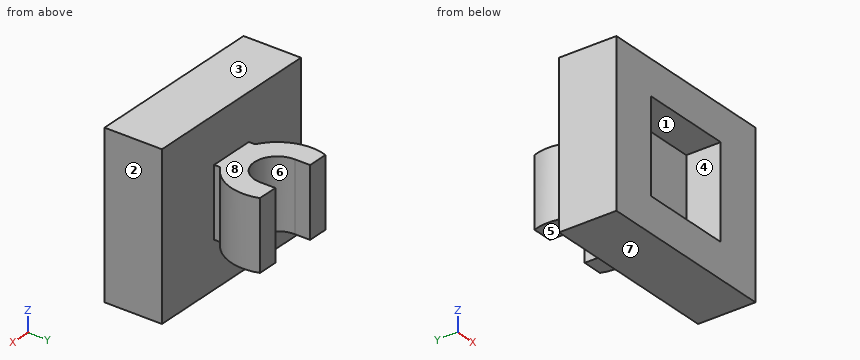
```python
from build123d import *

# Parameters (mm, degrees)
SKETCH1_W           = 10.16
SKETCH1_H           = 3.175
BOSS_EXTRUDE1_DEPTH = 4.445
BOSS_EXTRUDE2_DEPTH = 1.905
SKETCH3_OUTSIDE_W   = 15.162
SKETCH3_OUTSIDE_H   = 13.892
SKETCH3_OUTSIDE_W_2 = 10.16
SKETCH3_OUTSIDE_H_2 = 8.89
SKETCH3_OUTSIDE_W_3 = 5.08
SKETCH3_OUTSIDE_H_3 = 5.08
CUT_EXTRUDE1_DEPTH  = 1.905


with BuildPart() as part:
    # Sketch1 → Boss-Extrude1 (new body, symmetric)
    with BuildSketch(Plane.XY):
        with Locations((0, -1.5875)):
            Rectangle(SKETCH1_W, SKETCH1_H)
    extrude(amount=BOSS_EXTRUDE1_DEPTH, both=True)

    # Sketch2 → Boss-Extrude2 (add, symmetric)
    with BuildSketch(Plane.XY):
        with BuildLine():
            Line((-1.27, 2.54), (-1.27, 3.386666667))
            Line((-1.27, 3.386666667), (-2.394734966, 3.386666667))
            ThreePointArc((-2.394734966, 3.386666667), (-2.382785125, 1.660264217), (-1.27, 0.340295474))
            Line((-1.27, 0.340295474), (-1.27, 0))
            Line((-1.27, 0), (1.27, 0))
            Line((1.27, 0), (1.27, 0.340295474))
            ThreePointArc((1.27, 0.340295474), (2.382785125, 1.660264217), (2.394734966, 3.386666667))
            Line((2.394734966, 3.386666667), (1.27, 3.386666667))
            Line((1.27, 3.386666667), (1.27, 2.54))
            ThreePointArc((1.27, 2.54), (0, 1.27), (-1.27, 2.54))
        make_face()
    extrude(amount=BOSS_EXTRUDE2_DEPTH, both=True)

    # Sketch3 outside → Cut-Extrude1 (cut)
    with BuildSketch(Plane.XZ.offset(3.175)):
        Rectangle(SKETCH3_OUTSIDE_W, SKETCH3_OUTSIDE_H)
        Rectangle(SKETCH3_OUTSIDE_W_2, SKETCH3_OUTSIDE_H_2, mode=Mode.SUBTRACT)
        Rectangle(SKETCH3_OUTSIDE_W_3, SKETCH3_OUTSIDE_H_3)
    extrude(amount=-CUT_EXTRUDE1_DEPTH, mode=Mode.SUBTRACT)


solid = part.part
```
Can you work these out from the model? Positions are in its coordinate system, mm. Face numbers are marked on the shaded views. A direction names the side the tool comes from. Round coordinates to 2 decimals unless told otherwise and drop trailing zeros. Loops run counter-clockwise (first coordinate to the right, second up) from the corner with the lowest first, then second, coordinate; pieces in that order, holes last. Notation, with made-up numbers: (-8.75, -18) -> (31.25, -18) arc R19 cw to (31.25, -6) -> close; hole circle Ø5 at (79.25, 43). An arc over 180 degrees is marked (long way). Answer in a Markdown table with one row per item.
Item 1: Suppose I cut it at D-D, the plane y = 2.75. List the corners of the cut face in (x, z) for me (3 decimals).
Answer block:
| item | result |
|---|---|
| outline | (-2.531, -1.905) -> (-1.27, -1.905) -> (-1.27, 1.905) -> (-2.531, 1.905) -> close; (1.27, -1.905) -> (2.531, -1.905) -> (2.531, 1.905) -> (1.27, 1.905) -> close |
Item 2: We'd pull the mould along X, two halves only. Please class the marked faces 1, 2 and 3: released by +X, released by -X, zero draft, split by the parting line, or undercut.
Answer block:
| item | result |
|---|---|
| face 1 | undercut |
| face 2 | released by +X |
| face 3 | zero draft |
Item 3: If I drill on probe 1 along Z at (x, y) = (-1.75, -1.75) (3 decimals); probe 2 along X at (y, z) = (-1.75, 0.75); probe 3 along Y at (x, z) = (0.25, -2.75) (3 decimals), over which ranges is the centre line in solid material (lowest first)?
Answer block:
| item | result |
|---|---|
| probe 1 | -4.445 to -2.54, 2.54 to 4.445 |
| probe 2 | -5.08 to -2.54, 2.54 to 5.08 |
| probe 3 | -3.175 to 0 |
Item 4: Will these pins go through, and if not, where does the flat tip stop? P1, Ø5, axis at x = 1, z = -2.5, coming from the -Y side (3 decimals); P2, Ø1, axis at x = 1.5, z = -0.5, coming from the -Y side; P3, Ø1, axis at x = 0.5, y = 1, coming from the +Z side (3 decimals); P4, Ø0.7, axis at y = 3, z = -1, coming from the +X side.
Answer block:
| item | result |
|---|---|
| P1 | y = -3.175 |
| P2 | y = -1.27 |
| P3 | z = 1.905 |
| P4 | x = 2.54 |
Item 5: Suppose I cut it at A-A, the plane y = -2.5. List the corners of the cut face in (x, z) for me (3 decimals), plus the area to 3 significant figures.
Answer block:
| item | result |
|---|---|
| outline | (-5.08, -4.445) -> (5.08, -4.445) -> (5.08, 4.445) -> (-5.08, 4.445) -> close; hole (-2.54, -2.54) -> (2.54, -2.54) -> (2.54, 2.54) -> (-2.54, 2.54) -> close |
| area | 64.5 mm² |
Item 6: Suppose I cut it at C-C, the plane z = -0.75. List the corners of the cut face in (x, y) for me (3 decimals).
Answer block:
| item | result |
|---|---|
| outline | (-5.08, -3.175) -> (-2.54, -3.175) -> (-2.54, -1.27) -> (2.54, -1.27) -> (2.54, -3.175) -> (5.08, -3.175) -> (5.08, 0) -> (1.27, 0) -> (1.27, 0.34) arc R2.54 ccw to (2.395, 3.387) -> (1.27, 3.387) -> (1.27, 2.54) arc R1.27 cw to (-1.27, 2.54) -> (-1.27, 3.387) -> (-2.395, 3.387) arc R2.54 ccw to (-1.27, 0.34) -> (-1.27, 0) -> (-5.08, 0) -> close |
Item 7: On a 3-axis mill with a long thin cutter (end or side, diameter ignored), from which of +Z, -Z, +X, -X, +Y, -Y can I reach the whole of each face in a straight line? I mean the marked faces 4, 5, 6, 7 and 8. Say none if no direction works.
Answer block:
| item | result |
|---|---|
| face 4 | -Y |
| face 5 | -Z, +X, -X, +Y |
| face 6 | +Z, -Z, +Y |
| face 7 | -Z, +X, -X, +Y, -Y |
| face 8 | +Z, +X, -X, +Y |
Item 8: Suppose I cut it at B-B, the plane x = 0. List the corners of the cut face in (y, z) for me (3 decimals), plus the area to 3 significant figures.
Answer block:
| item | result |
|---|---|
| outline | (-3.175, -4.445) -> (0, -4.445) -> (0, -1.905) -> (1.27, -1.905) -> (1.27, 1.905) -> (0, 1.905) -> (0, 4.445) -> (-3.175, 4.445) -> (-3.175, 2.54) -> (-1.27, 2.54) -> (-1.27, -2.54) -> (-3.175, -2.54) -> close |
| area | 23.4 mm² |
